```python
from build123d import *

# Parameters (mm, degrees)
SKETCH001_R             = 0.75
PAD_DEPTH               = 10
POCKET001_DEPTH         = 5
POCKET002_DEPTH         = 2
BODY001_ROLL_ANGLE      = 44.999986
BODY001_PITCH_ANGLE     = -3.6e-05
BODY001_PLACEMENT_ANGLE = -44.999986


with BuildPart() as part:
    # Sketch001 → Pad (new body)
    with BuildSketch(Plane.XY):
        Polygon((-26.02, -9.66), (28.45, -9.66), (28.45, 9.34), (22.45, 9.34), (22.45, 1.34), (10.95, 1.34), (10.95, 9.34), (-26.02, 9.34), align=None)
        with Locations((-24.19, 7.43)):
            Circle(SKETCH001_R, mode=Mode.SUBTRACT)
        with Locations((25.81, 0)):
            Circle(SKETCH001_R, mode=Mode.SUBTRACT)
    extrude(amount=PAD_DEPTH)

    # Sketch007 → Pocket001 (cut)
    with BuildSketch(Plane.XY):
        with BuildLine():
            Line((-26.02, -9.66), (-26.02, 9.34))
            Line((-26.02, 9.34), (28.45, 9.34))
            Line((28.45, 9.34), (28.45, -9.66))
            Line((27.21, -9.66), (28.45, -9.66))
            Line((27.21, -9.66), (27.21, 0))
            ThreePointArc((27.21, 0), (25.81, 1.4), (24.41, 0))
            Line((24.41, 0), (24.41, -9.66))
            Line((-22.79, -9.66), (24.41, -9.66))
            Line((-22.79, -9.66), (-22.79, 7.43))
            ThreePointArc((-22.79, 7.43), (-24.19, 8.83), (-25.59, 7.43))
            Line((-25.59, 7.43), (-25.59, -9.66))
            Line((-26.02, -9.66), (-25.59, -9.66))
        make_face()
    extrude(amount=-POCKET001_DEPTH, mode=Mode.SUBTRACT)

    # Sketch007 → Pocket002 (cut)
    with BuildSketch(Plane.XY):
        with BuildLine():
            Line((-26.02, -9.66), (-26.02, 9.34))
            Line((-26.02, 9.34), (28.45, 9.34))
            Line((28.45, 9.34), (28.45, -9.66))
            Line((27.21, -9.66), (28.45, -9.66))
            Line((27.21, -9.66), (27.21, 0))
            ThreePointArc((27.21, 0), (25.81, 1.4), (24.41, 0))
            Line((24.41, 0), (24.41, -9.66))
            Line((-22.79, -9.66), (24.41, -9.66))
            Line((-22.79, -9.66), (-22.79, 7.43))
            ThreePointArc((-22.79, 7.43), (-24.19, 8.83), (-25.59, 7.43))
            Line((-25.59, 7.43), (-25.59, -9.66))
            Line((-26.02, -9.66), (-25.59, -9.66))
        make_face()
    extrude(amount=POCKET002_DEPTH, mode=Mode.SUBTRACT)


with BuildPart() as part_1:
    # Body001 roll: moved
    add(part.part.rotate(Axis((0, 0, 0), (1, 0, 0)), BODY001_ROLL_ANGLE))


with BuildPart() as part_2:
    # Body001 pitch: moved
    add(part_1.part.rotate(Axis((0, 0, 0), (0, 1, 0)), BODY001_PITCH_ANGLE))


with BuildPart() as part_3:
    # Body001 placement: moved
    add(part_2.part.moved(Location((25.88, 22.93, 6.87071))).rotate(Axis((25.88, 22.93, 6.87071), (0, 0, 1)), BODY001_PLACEMENT_ANGLE))


solid = part_3.part
```
Part model, mm, in its own coordinate system. A direction names the side the tool comes from. Round coordinates to 2 decimals unless told otherwise and drop trailing zeros. Write each loop counter-clockwise with the first axis right and the second up, starting at its lowest first coordinate (ties: lowest second). Pieces come first, ordered by that corner, then holes. Notation, with made-up numbers: (32, 21) -> (87, 21) arc R21 cw to (87, 50) -> close; hole circle Ø5 at (80, 18). An arc over 180 degrees is marked (long way). Return JSON: item names as keys, results as strings. Group by question number.
Q1. Saw through at D-D on x = 17.5. Write the cut outline in (y, z).
Q2. Probe L1, parallel to X at y = 8, z = 12.5; L2, parallel to X at y = 1, z = 11.5; L3, parallel to X at y = 27, z = 2. List the from-to ranges inside material, lowest first. Write a range as [from, to].
Q3. Mould opens along Y. For faces 1 (the flat face through (18.62, 14.49, 4.31)), 2 (the flat face through (35.444, 8.762, 12.021)), 3 (the flat face through (41.5, 6.8, 14.9)) say: pulls with the +Y half, pulls with the -Y half, needs draft (parallel to the pull), parting line crosses it, or undercut.
Q4. Saw through at C-C on z = 2.25. Write the cut outline in (x, y), plus the area to 3 significant figures.
Q5. Which spindle directions (+Z, -Z, +X, -X, +Y, -Y) get a long thin tool onto all of the face, cutting with end or side? Do faces 4 (the flat face through (33.293, 14.857, 14.81)), 5 (the flat face through (8.65, 37.93, 6.69)), 6 (the cylindrical face through (12.719, 43.935, 13.811)), 7 (the flat face through (40.27, 2.8, 4.2)). Say none if no direction does.
Q6. Pin check, flat tips, straight feed: pin 1 (2 mm diameter, centred on y = 10.5, z = 12.5, fed in from -X); pin 2 (12 mm diameter, centred on x = 16, y = 16, fed in from +Z); pin 3 (1.5 mm diameter, centred on x = 43, z = 2, fed in from +Y); pin 4 (5 mm diameter, centred on y = 8.5, z = 10.5, fed in from +X). Stop position of each tip, or through.
Q7. Saw through at A-A on z = 17. State how many separate pieces and enclosed holes the cut face has, plus the area to 3 significant figures.
Q8. Saw through at B-B on y = 16.5. Write the cut outline in (x, z).
Answer:
{
 "1": {"outline": "(11.65, 7.11) -> (19.65, 1.45) -> (38.65, 14.89) -> (30.65, 20.55) -> close"},
 "2": {"L1": "[28.77, 35.53], [42.7, 44.77]", "L2": "[34.36, 39.94], [41.5, 44.18]", "L3": "[9.38, 10.92]"},
 "3": {"face 1": "pulls with the -Y half", "face 2": "undercut", "face 3": "pulls with the +Y half"},
 "4": {"outline": "(1.09, 34.94) -> (39.6, -3.58) -> (40.73, -2.45) -> (39.85, -1.58) -> (41.85, 0.42) -> (39.87, 2.4) -> (37.87, 0.4) -> (4.5, 33.78) -> (6.5, 35.78) -> (4.52, 37.76) -> (2.52, 35.76) -> (2.21, 36.06) -> close", "area": "103 mm2"},
 "5": {"face 4": "+Z, +X", "face 5": "-Z, +X", "face 6": "none", "face 7": "-Z, +Y"},
 "6": {"pin 1": "x = 24.54", "pin 2": "z = 15.13", "pin 3": "through", "pin 4": "x = 45.77"},
 "7": {"separate pieces": "2", "enclosed holes": "1", "area": "302 mm2"},
 "8": {"outline": "(12.65, 7.11) -> (20.65, 1.45) -> (34.94, 11.56) -> (34.94, 18.22) -> (31.65, 20.55) -> close"}
}
